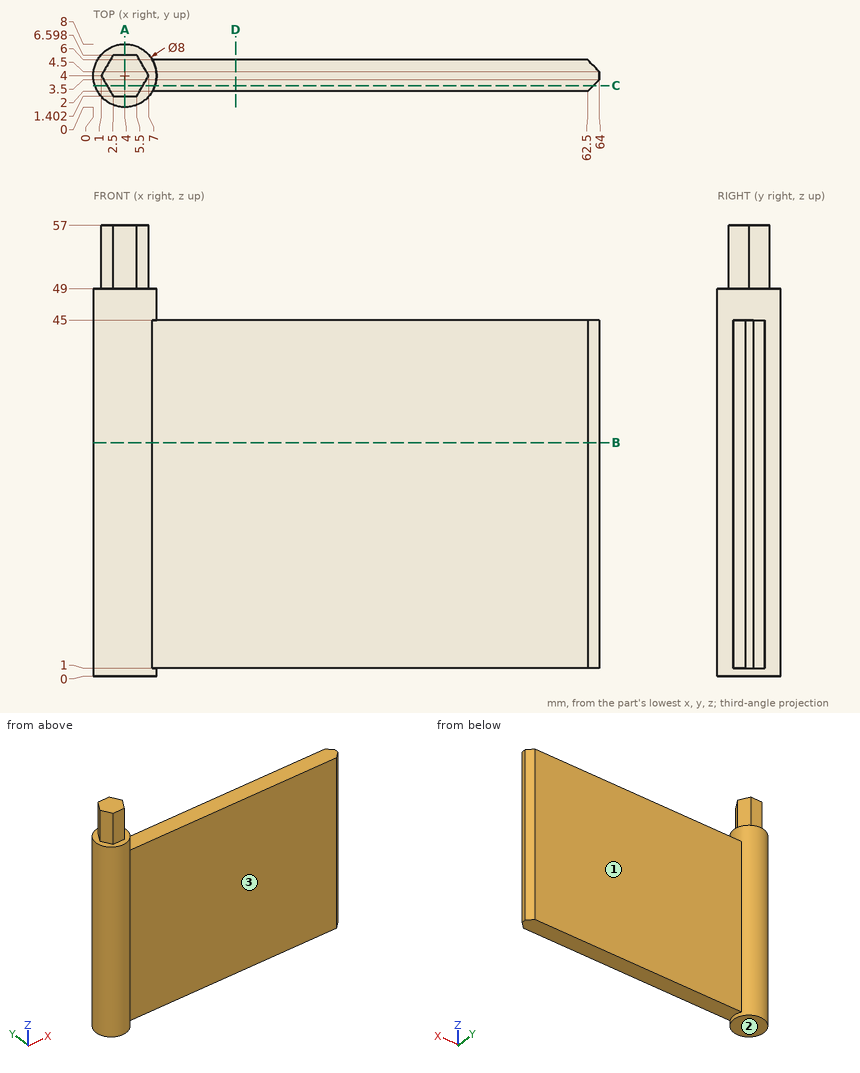
The drawing under review shows one solid part. Ordinate dimensions are in mm from its lowest x, y, z. A direction names the side the tool comes from. Round coordinates to 2 decimals unless told otherwise and drop trailing zeros. Write each loop counter-clockwise with the first axis right and the second up, starting at its lowest first coordinate (ties: lowest second). Pieces come first, ordered by that corner, then holes. Notation, with made-up numbers: (17, 18) - (49, 18) arc R31 cw to (49, 57) - close; hole circle Ø7 at (80, -37). An arc over 180 degrees is marked (long way). Use a Markdown table: item, result. Add a question column.
1. For the marked faces 1, 2 and 3, list the 3-axis set-ups (+Z, -Z, +X, -X, +Y, -Y) from which the entire face can be reached by the end or side of a thin tool; tool diameter is ignored.
2. Clearance check with flat-ended pins moving along their axes: pin 1 (2 mm diameter, centred on x = 25.5, y = 3.5, fed in from -Z); pin 2 (3 mm diameter, centred on x = 37, y = 4.5, fed in from +Z); pin 3 (22 mm diameter, centred on x = 40.5, z = 28, fed in from +Y). State where each tip first meets the part, or that it passes through.
3. Wall thickness on probe 1 along Y at (x, z) = (40, 13); probe 2 along Z at (x, y) = (23.5, 5.25); probe 3 along X at (y, z) = (3.75, 43): over which ranges is each line inside the solid? List them lowest first.
4. We need section D-D (x = 18). State the section outline as (y, z) points.
5. We need section A-A (x = 4). State the section outline as (y, z) points.
6. We need section B-B (z = 29.5). State the section outline as (x, y) points.
7. We need section C-C (y = 2.75). State the section outline as (x, z) points.
Output:
| question | item | result |
|---|---|---|
| 1 | face 1 | +Z, -Z, +X, +Y |
| 1 | face 2 | -Z, +X, -X, +Y, -Y |
| 1 | face 3 | +Z, -Z, +X, -Y |
| 2 | pin 1 | stops at z = 1 |
| 2 | pin 2 | stops at z = 45 |
| 2 | pin 3 | stops at y = 6 |
| 3 | probe 1 | y = 2 to 6 |
| 3 | probe 2 | z = 1 to 45 |
| 3 | probe 3 | x = 0.01 to 64 |
| 4 | outline | (2, 1) - (6, 1) - (6, 45) - (2, 45) - close |
| 5 | outline | (0, 0) - (8, 0) - (8, 49) - (6.6, 49) - (6.6, 57) - (1.4, 57) - (1.4, 49) - (0, 49) - close |
| 6 | outline | (7.46, 2) - (62.5, 2) - (64, 3.5) - (64, 4.5) - (62.5, 6) - (7.46, 6) arc R4 ccw (long way) to start |
| 7 | outline | (0.2, 0) - (7.8, 0) - (7.8, 1) - (63.25, 1) - (63.25, 45) - (7.8, 45) - (7.8, 49) - (6.28, 49) - (6.28, 57) - (1.72, 57) - (1.72, 49) - (0.2, 49) - close |
